from build123d import *

# Parameters (mm, degrees)
SKETCH_1_W          = 78
SKETCH_1_H          = 42
EXTRUDE_1_DEPTH     = 25
SHELL_1_T           = 1
SKETCH_2_W          = 90
SKETCH_2_H          = 55
SKETCH_2_W_2        = 80
SKETCH_2_H_2        = 44
EXTRUDE_2_DEPTH     = 1
SKETCH_3_W          = 5
SKETCH_3_H          = 44
CUT_EXTRUDE_1_DEPTH = 5


with BuildPart() as part:
    # 草图1 → 凸台-拉伸1 (new body)
    with BuildSketch(Plane(origin=(0, 0, 0), x_dir=(1, 0, 0), z_dir=(0, 1, 0))):
        Rectangle(SKETCH_1_W, SKETCH_1_H)
    extrude(amount=EXTRUDE_1_DEPTH)

    # 抽壳1
    shell_1_openings = [part.faces().sort_by_distance(p)[0] for p in [
        (0, 0, 0),
    ]]
    offset(amount=SHELL_1_T, openings=shell_1_openings, kind=Kind.INTERSECTION)

    # 草图2 → 凸台-拉伸2 (add)
    with BuildSketch(Plane.XZ):
        Rectangle(SKETCH_2_W, SKETCH_2_H)
        Rectangle(SKETCH_2_W_2, SKETCH_2_H_2, mode=Mode.SUBTRACT)
    extrude(amount=-EXTRUDE_2_DEPTH)

    # 草图3 → 切除-拉伸1 (cut)
    with BuildSketch(Plane(origin=(0, 26, 0), x_dir=(1, 0, 0), z_dir=(0, 1, 0))):
        with Locations((-37.5, 0)):
            Rectangle(SKETCH_3_W, SKETCH_3_H)
        with Locations((37.5, 0)):
            Rectangle(SKETCH_3_W, SKETCH_3_H)
    extrude(amount=-CUT_EXTRUDE_1_DEPTH, mode=Mode.SUBTRACT)


solid = part.part
Source: CAD feature listing. Evaluate the final solid. Frame: model axes, mm. A direction names the side the tool comes from. Round coordinates to 2 decimals unless told otherwise and drop trailing zeros. Loops run counter-clockwise (first coordinate to the right, second up) from the corner with the lowest first, then second, coordinate; pieces in that order, holes last. Notation, with made-up numbers: M 21,-33.5 L 42,-33.5 A18 ccw 42,-16.5 Z; hole C 46.25,-1 d6. An arc over 180 degrees is marked long. Return JSON: item names as keys, results as strings. Group by question number.
1. Section query C-C on x = 28.5. Output: boundary loops of the cut face in (y, z), and give its area (3 significant figures).
2. Reachability of faces 1 (the face through (-1, 13, -22)), 2 (the face through (39, 10, 0)), 3 (the face through (-1, 12, 21)), 4 (the face through (-1, 13, 22)) from +Z, -Z, +X, -X, +Y, -Y: full face, straight path, thin tool, end or side. Return the list, or none.
3. Material intervals for line 1 along Z through (x, y) = (-12.5, 16.25); line 2 along X through (y, z) = (8.75, -18); line 3 along Y through (x, z) = (-28.5, -19), sorted ascending. Write a range as from..to.
4. Mould query, pull axis X, two halves, no side actions, for faces 5 (the face through (-39, 10, 0)), 6 (the face through (-1, 0, -24)), 7 (the face through (-35, 25.4, 0.1)), 8 (the face through (35, 25.4, 0.1)). Classes: released by +X, released by -X, zero draft, split by the parting line, or undercut.
5. Pin query (flat end, axial travel): pin 1 (10.5 mm diameter, centred on y = 14, z = -4, fed in from +X); pin 2 (1 mm diameter, centred on x = 13, y = 15, fed in from +Z); pin 3 (3 mm diameter, centred on x = 30, y = 6, fed in from -Z). Return the tip coordinate at first contact, or that it passes through.
6. Section query D-D on z = 23. Output: boundary loops of the cut face in (x, y), and give its area (3 significant figures).
7. Section query B-B on y = 12.25. Output: boundary loops of the cut face in (x, z).
8. Section query A-A on z = 5. Output: boundary loops of the cut face in (x, y).
Checks:
{
 "1": {"outline": "M 0,-27.5 L 1,-27.5 L 1,-22 L 26,-22 L 26,22 L 1,22 L 1,27.5 L 0,27.5 L 0,21 L 25,21 L 25,-21 L 0,-21 Z", "area": "105 mm²"},
 "2": {"face 1": "-Z, +X, -X, +Y", "face 2": "+Y, -Y", "face 3": "-Y", "face 4": "+Z, +X, -X, +Y"},
 "3": {"line 1": "z = -22..-21, 21..22", "line 2": "x = -40..-39, 39..40", "line 3": "y = 25..26"},
 "4": {"face 5": "undercut", "face 6": "zero draft", "face 7": "released by -X", "face 8": "released by +X"},
 "5": {"pin 1": "stops at x = 40", "pin 2": "stops at z = 22", "pin 3": "stops at z = -22"},
 "6": {"outline": "M -45,0 L 45,0 L 45,1 L -45,1 Z", "area": "90.0 mm²"},
 "7": {"outline": "M -40,-22 L 40,-22 L 40,22 L -40,22 Z; hole M -39,-21 L 39,-21 L 39,21 L -39,21 Z"},
 "8": {"outline": "M -45,0 L -39,0 L -39,21 L -40,21 L -40,1 L -45,1 Z; M -35,25 L 35,25 L 35,26 L -35,26 Z; M 39,0 L 45,0 L 45,1 L 40,1 L 40,21 L 39,21 Z"}
}
